from build123d import *

# Parameters (mm, degrees)
F0_R     = 3
F0_R_2   = 5
F1_DEPTH = 5


with BuildPart() as f1:
    # F0 (on Front) → F1 (new body)
    with BuildSketch(Plane.XZ):
        with BuildLine():
            Line((-6.190103, 23.645651), (-63.179695, 23.645651))
            ThreePointArc((-63.179695, 23.645651), (-72.141327, 17.657681), (-70.038631, 7.086716))
            Line((-70.038631, 7.086716), (-56.597567, -6.354349))
            Line((-56.597567, -6.354349), (28.820305, -6.354349))
            Line((28.820305, -6.354349), (28.820305, -29.554349))
            Line((28.820305, -29.554349), (41.820305, -29.554349))
            Line((41.820305, -29.554349), (41.820305, 1.645651))
            Line((41.820305, 1.645651), (51.820305, 1.645651))
            Line((51.820305, 1.645651), (51.820305, 9.395651))
            Line((51.820305, 9.395651), (37.820305, 9.395651))
            ThreePointArc((37.820305, 9.395651), (33.570305, 13.645651), (37.820305, 17.895651))
            Line((37.820305, 17.895651), (51.820305, 17.895651))
            Line((51.820305, 17.895651), (51.820305, 23.645651))
            Line((51.820305, 23.645651), (16.653307, 23.645651))
            Line((16.653307, 23.645651), (16.080297, 23.645651))
            Line((16.080297, 23.645651), (5.830712, 23.645651))
            Line((5.830712, 23.645651), (12.825509, 16.650855))
            ThreePointArc((12.825509, 16.650855), (12.825509, 10.640448), (6.815101, 10.640448))
            Line((6.815101, 10.640448), (-6.190103, 23.645651))
        make_face()
        with Locations((33.820305, -19.554349)):
            Circle(F0_R, mode=Mode.SUBTRACT)
        with Locations((-41.179695, 0.445651)):
            Circle(F0_R, mode=Mode.SUBTRACT)
        with Locations((-11.179695, 0.445651)):
            Circle(F0_R, mode=Mode.SUBTRACT)
        with Locations((-63.179695, 13.945651)):
            Circle(F0_R_2, mode=Mode.SUBTRACT)
        with Locations((18.820305, 0.445651)):
            Circle(F0_R, mode=Mode.SUBTRACT)
    extrude(amount=F1_DEPTH)


solid = f1.part
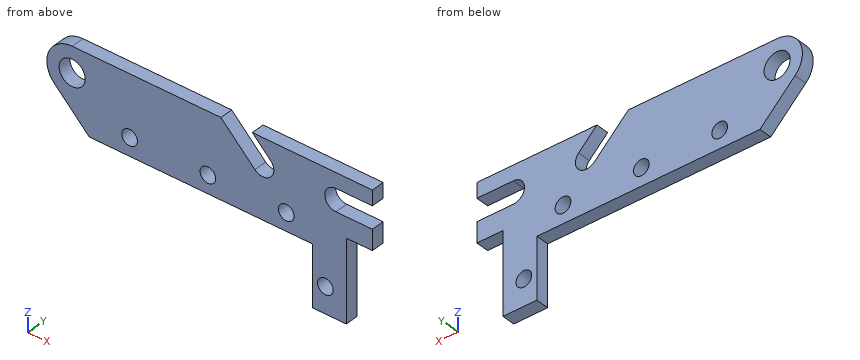
Work out the finished part from the listing and answer in its coordinate system (mm). Give positions to 0.01 mm unless a question says otherwise; leave off trailing zeros. Loops run counter-clockwise (first coordinate to the right, second up) from the corner with the lowest first, then second, coordinate; pieces in that order, holes last. Notation, with made-up numbers: (13, 47) - (21, 47) arc R23 ccw to (21, 60) - close; hole circle Ø3 at (49.5, -11). An arc over 180 degrees is marked (long way). Answer in a Markdown table with one row per item.
(1) Consider L1, parallel to X at y = -2.7, z = 1; L2, parallel to X at y = -3.2, z = 1.5; L3, parallel to Z at x = -22, y = -3.5. Determine where each line is inside the solid, lowest interval first. Write a range as [from, to].
Results list:
| item | result |
|---|---|
| L1 | x = [-63.95, -44.13], [-38.23, -14.13], [-8.23, 15.87], [21.77, 41.82] |
| L2 | x = [-64.45, -43.99], [-38.37, -13.99], [-8.37, 16.01], [21.63, 41.82] |
| L3 | z = [-6.35, 23.65] |
(2) Section B-B (y = -3.55) is taken. Give the vertices of the cut face in (x, z).
Results list:
| item | result |
|---|---|
| outline | (-70.04, 7.09) - (-56.6, -6.35) - (28.82, -6.35) - (28.82, -29.55) - (41.82, -29.55) - (41.82, 1.65) - (51.82, 1.65) - (51.82, 9.4) - (37.82, 9.4) arc R4.25 cw to (37.82, 17.9) - (51.82, 17.9) - (51.82, 23.65) - (5.83, 23.65) - (12.83, 16.65) arc R4.25 cw to (6.82, 10.64) - (-6.19, 23.65) - (-63.18, 23.65) arc R9.7 ccw to start; hole circle Ø10 at (-63.18, 13.95); hole circle Ø6 at (-41.18, 0.45); hole circle Ø6 at (-11.18, 0.45); hole circle Ø6 at (18.82, 0.45); hole circle Ø6 at (33.82, -19.55) |
(3) Section D-D (x = -18) is taken. Give the vertices of the cut face in (y, z), and give its area (3 significant figures).
Results list:
| item | result |
|---|---|
| outline | (-5, -6.35) - (0, -6.35) - (0, 23.65) - (-5, 23.65) - close |
| area | 150 mm² |
(4) Flat-ended cylindrical pins translate along their axes: pin 1 Ø5.5 at (x, z) = (-11.18, 0.45) entering from -Y; pin 2 Ø1.5 at (x, y) = (46, -3) entering from -Z; pin 3 Ø1.5 at (y, z) = (-1.5, -23.5) entering from -X; pin 4 Ø1.5 at (x, y) = (-19, -3) entering from -Z. Find the tip coordinate at first contact, or state that the pin passes through.
Results list:
| item | result |
|---|---|
| pin 1 | passes through |
| pin 2 | stops at z = 1.65 |
| pin 3 | stops at x = 28.82 |
| pin 4 | stops at z = -6.35 |
(5) Section C-C (z = -11) is taken. Give the vertices of the cut face in (x, y), and give its area (3 significant figures).
Results list:
| item | result |
|---|---|
| outline | (28.82, -5) - (41.82, -5) - (41.82, 0) - (28.82, 0) - close |
| area | 65.0 mm² |
(6) Section A-A (x = 19.5) is taken. Give the vertices of the cut face in (y, z).
Results list:
| item | result |
|---|---|
| outline | (-5, -6.35) - (0, -6.35) - (0, -2.48) - (-5, -2.48) - close; (-5, 3.37) - (0, 3.37) - (0, 23.65) - (-5, 23.65) - close |
